```python
from build123d import *

# Parameters (mm, degrees)
BOSS_EXTRUDE1_DEPTH      = 12.5
BOSS_EXTRUDE1_DEPTH_BACK = 12.5
F_10_0MM_DOWEL_HOLE1_D   = 10
FILLET1_R                = 2
SKETCH3_W                = 16
SKETCH3_H                = 30
BOSS_EXTRUDE2_DEPTH      = 10
BOSS_EXTRUDE3_DEPTH      = 10


with BuildPart() as part:
    # Sketch1 → Boss-Extrude1 (new, two sides: drawn at the far end of the back side and taken through both)
    with BuildSketch(Plane.XY.offset(-BOSS_EXTRUDE1_DEPTH_BACK)):
        Polygon((0, 0), (2, 0), (2, -63), (37, -63), (37, -98), (35, -98), (35, -65), (0, -65), align=None)
    extrude(amount=BOSS_EXTRUDE1_DEPTH + BOSS_EXTRUDE1_DEPTH_BACK)

    # Ø10.0mm Dowel Hole1 (through all)
    with Locations(Plane(origin=(2, -26, 0), x_dir=(0, 1, 0), z_dir=(1, 0, 0))):
        with Locations((0, 0)):
            Hole(F_10_0MM_DOWEL_HOLE1_D / 2)

    # Fillet1
    fillet1_edges = [part.edges().sort_by_distance(p)[0] for p in [
        (2, -63, 0),
        (37, -63, 0),
        (35, -65, 0),
        (0, -65, 0),
    ]]
    fillet(fillet1_edges, radius=FILLET1_R)

    # Sketch3 → Boss-Extrude2 (add)
    with BuildSketch(Plane(origin=(37, 0, 0), x_dir=(0, 0, -1), z_dir=(1, 0, 0))):
        with Locations((0, -82.60435288)):
            Rectangle(SKETCH3_W, SKETCH3_H)
    extrude(amount=BOSS_EXTRUDE2_DEPTH)

    # Sketch4 → Boss-Extrude3 (add)
    with BuildSketch(Plane(origin=(47, 0, 0), x_dir=(0, 0, -1), z_dir=(1, 0, 0))):
        Polygon((-8, -69.135252509), (-26.480043417, -94.242566668), (-26.046645408, -94.559298491), (-8, -69.410399443), align=None)
    extrude(amount=-BOSS_EXTRUDE3_DEPTH)


solid = part.part
```
Input: part model. Units: mm. Frame: model coordinates. A direction names the side the tool comes from. Give positions to 0.01 mm unless a question says otherwise; leave off trailing zeros. Loops run counter-clockwise (first coordinate to the right, second up) from the corner with the lowest first, then second, coordinate; pieces in that order, holes last.
1) Section query B-B on y = -26. Return the cut outline in (x, z).
A:
outline: (0, -12.5) - (2, -12.5) - (2, -5) - (0, -5) - close; (0, 5) - (2, 5) - (2, 12.5) - (0, 12.5) - close
2) Section query A-A on z = 0. Return the cut outline in (x, y), and give its area (3 significant figures).
A:
outline: (0, -63) arc R2 ccw to (2, -65) - (33, -65) arc R2 cw to (35, -67) - (35, -98) - (37, -98) - (37, -97.6) - (47, -97.6) - (47, -67.6) - (37, -67.6) - (37, -65) arc R2 ccw to (35, -63) - (4, -63) arc R2 cw to (2, -61) - (2, -31) - (0, -31) - close; (0, -21) - (2, -21) - (2, 0) - (0, 0) - close
area: 546 mm2
3) Section query D-D on x = 11. Return the cut outline in (y, z).
A:
outline: (-65, -12.5) - (-63, -12.5) - (-63, 12.5) - (-65, 12.5) - close
4) Contact query for flat-ended pins moving along their axis: pin 1 (3 mm diameter, centred on x = 42.5, y = -86, fed in from +Z); pin 2 (4 mm diameter, centred on y = -87, z = 20.5, fed in from -X); pin 3 (8 mm diameter, centred on x = 43.5, z = 1.5, fed in from -Y). Output: stop coordinate, or through.
A:
pin 1: stops at z = 21.52
pin 2: stops at x = 37
pin 3: stops at y = -97.6
5) Section query C-C on z = 6.5. Return the cut outline in (x, y), and give its area (3 significant figures).
A:
outline: (0, -63) arc R2 ccw to (2, -65) - (33, -65) arc R2 cw to (35, -67) - (35, -98) - (37, -98) - (37, -97.6) - (47, -97.6) - (47, -67.6) - (37, -67.6) - (37, -65) arc R2 ccw to (35, -63) - (4, -63) arc R2 cw to (2, -61) - (2, 0) - (0, 0) - close
area: 566 mm2
6) Reachability of faces 1 (the flat face through (2, -30, -6)), 2 (the flat face through (42.1, -81.5, 17.1)), 3 (the flat face through (35, -83, 0)), 4 (the flat face through (42, -97.604, 0)) from +Z, -Z, +X, -X, +Y, -Y: full face, straight path, thin tool, end or side. Return the list, or none.
A:
face 1: +Z, -Z, +X, +Y
face 2: +Z, +X, +Y
face 3: +Z, -Z, -X, -Y
face 4: +Z, -Z, +X, -Y
7) Line query: L1, parallel to Y at x = 28, z = -4.5; L2, parallel to X at y = -25, z = 8; L3, parallel to Z at x = 1, y = -26. Output: solid intervals per line, ascending.
A:
L1: y = -65 to -63
L2: x = 0 to 2
L3: z = -12.5 to -5, 5 to 12.5
8) Mould query, pull axis Z, two halves, no side actions, for faces 5 (the flat face through (19, -63, 0)), 6 (the flat face through (42, -84, 8)), 7 (the flat face through (42, -83, -8)), 8 (the flat face through (37, -81, -9)). Classes: released by +Z, released by -Z, zero draft, split by the parting line, or undercut.
A:
face 5: zero draft
face 6: undercut
face 7: released by -Z
face 8: undercut
